Design review of the part built by this model. Coordinates are the model's own, in mm. Face numbers are marked on the shaded views. A direction names the side the tool comes from. Round coordinates to 2 decimals unless told otherwise and drop trailing zeros. Order: outer loops, then holes, each group sorted by start corner. A loop starts at its lowest first (then second) coordinate and runs counter-clockwise, first axis right, second up. Notation, with made-up numbers: M 6.25,74 L 24.25,74 A22 cw 24.25,85 Z; hole C 9,55 d9. An arc over 180 degrees is marked long. Use a Markdown table: item, result. Add a question column.
(1) For pin 1 (6 mm diameter, centred on x = -10.5, z = 10, fed in from +Y); pin 2 (12 mm diameter, centred on x = 8.5, z = 25, fed in from -Y); pin 3 (2.5 mm diameter, centred on x = 0, y = 12.75, fed in from -Z); pin 4 (1.5 mm diameter, centred on y = 1, z = 15, fed in from +X), all flat-tipped, find the tip position at first contact; note any pin that passes through.
(2) To check wall thickness, follow probe 1 along Z at (x, y) = (-12, 7.25); probe 2 along Y at (x, z) = (0, 6.5); probe 3 along Y at (x, z) = (0, 18). State the ranges of each line that lie inside material, in increasing order. Write a range as from..to.
(3) Machinability: for the marked faces 1, 2, 3 and 4, which of the approach directions +Z, -Z, +X, -X, +Y, -Y give a long, thin tool a straight path to every point of the face, cutting with its end or side? Answer none if there is none.
(4) Take a section at A-A (z = 29). Write out the cut boundary in (x, y), then the cut area to 3 significant figures.
(5) The part is to be moulded in two halves that separate along X. For the marked faces 5, 6, 7 and 8, say which applies: released by +X, released by -X, zero draft, split by the parting line, or undercut.
(6) Take a section at B-B (z = 20). Write out the cut boundary in (x, y).
```python
from build123d import *

# Parameters (mm, degrees)
ESQUISSE1_R                       = 14.25
BOSS_EXTRU_1_DEPTH                = 4
ESQUISSE2_R                       = 15
BOSS_EXTRU_2_DEPTH                = 28.5
ESQUISSE3_R                       = 12.5
BOSS_EXTRU_3_DEPTH                = 0.5
ESQUISSE4_R                       = 13
BOSS_EXTRU_4_DEPTH                = 5.25
DIAM_TRE_DU_PER_AGE_2_0_2_1_D     = 2
DIAM_TRE_DU_PER_AGE_2_0_2_1_DEPTH = 9
DIAM_TRE_DU_PER_AGE_2_0_2_1_TIP   = 0.600860619


with BuildPart() as part:
    # Esquisse1 → Boss.-Extru.1 (new body)
    with BuildSketch(Plane.XY):
        Circle(ESQUISSE1_R)
    extrude(amount=BOSS_EXTRU_1_DEPTH)

    # Esquisse2 → Boss.-Extru.2 (add)
    with BuildSketch(Plane.XY.offset(4)):
        with Locations(Location((0, 0, 0), (0, 0, 180))):
            Circle(ESQUISSE2_R)
    extrude(amount=BOSS_EXTRU_2_DEPTH)

    # Esquisse3 → Boss.-Extru.3 (add)
    with BuildSketch(Plane.XY.offset(32.5)):
        Circle(ESQUISSE3_R)
    extrude(amount=BOSS_EXTRU_3_DEPTH)

    # Esquisse4 → Boss.-Extru.4 (add)
    with BuildSketch(Plane.XY.offset(33)):
        with Locations(Location((0, 0, 0), (0, 0, 180))):
            Circle(ESQUISSE4_R)
    extrude(amount=BOSS_EXTRU_4_DEPTH)

    # Esquisse5 → Enlèvement de matière-Révolution1 (revolve, cut)
    with BuildSketch(Plane(origin=(0, 0, 0), x_dir=(0, 0, -1), z_dir=(1, 0, 0)), mode=Mode.PRIVATE) as enl_vement_de_mati_re_r_volution1_sk:
        Polygon((0, 0), (-38.25, 0), (-38.25, 11), (-32.75, 11), (-32.75, 9.75), (0, 9.75), align=None)
        with BuildLine():
            Line((-28, 15), (-12, 15))
            Line((-12, 15), (-12, 13.5))
            ThreePointArc((-12, 13.5), (-12.146446609, 13.146446609), (-12.5, 13))
            Line((-12.5, 13), (-27.5, 13))
            ThreePointArc((-27.5, 13), (-27.853553391, 13.146446609), (-28, 13.5))
            Line((-28, 13.5), (-28, 15))
        make_face()
    revolve(enl_vement_de_mati_re_r_volution1_sk.sketch.rotate(Axis((0, 0, 0), (0, 0, 1)), 90), axis=Axis((0, 0, 0), (0, 0, 1)), mode=Mode.SUBTRACT)

    # Diamètre du perçage Ø2.0 (2)1
    with Locations(Plane(origin=(0, 0, 0), x_dir=(-1, 0, 0), z_dir=(0, 0, -1))):
        with Locations((0, 12.75)):
            Hole(DIAM_TRE_DU_PER_AGE_2_0_2_1_D / 2, depth=DIAM_TRE_DU_PER_AGE_2_0_2_1_DEPTH)
            with Locations((0, 0, -(DIAM_TRE_DU_PER_AGE_2_0_2_1_DEPTH + DIAM_TRE_DU_PER_AGE_2_0_2_1_TIP / 2))):  # 118° drill point
                Cone(0, DIAM_TRE_DU_PER_AGE_2_0_2_1_D / 2, DIAM_TRE_DU_PER_AGE_2_0_2_1_TIP, mode=Mode.SUBTRACT)


solid = part.part
```
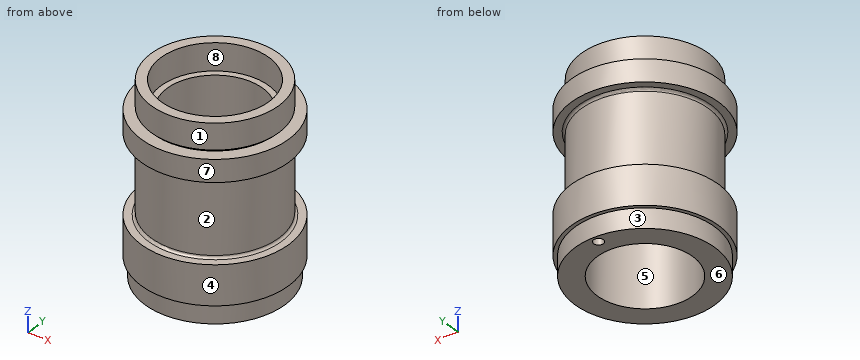
Verdict:
| question | item | result |
|---|---|---|
| 1 | pin 1 | stops at y = 12.99 |
| 1 | pin 2 | stops at y = -14.63 |
| 1 | pin 3 | stops at z = 0 |
| 1 | pin 4 | stops at x = 13 |
| 2 | probe 1 | z = 0..12, 28..32.5 |
| 2 | probe 2 | y = -15..-9.75, 9.75..11.75, 13.75..15 |
| 2 | probe 3 | y = -13..-9.75, 9.75..13 |
| 3 | face 1 | +Z |
| 3 | face 2 | none |
| 3 | face 3 | -Z |
| 3 | face 4 | +Z, -Z |
| 4 | outline | C 0,0 d30; hole C 0,0 d19.5 |
| 4 | area | 408 mm^2 |
| 5 | face 5 | undercut |
| 5 | face 6 | zero draft |
| 5 | face 7 | split by the parting line |
| 5 | face 8 | undercut |
| 6 | outline | C 0,0 d26; hole C 0,0 d19.5 |
